Work out the finished part from the listing and answer in its coordinate system (mm). Face numbers are marked on the shaded views. A direction names the side the tool comes from. Coordinates: 2 decimals unless noted, no trailing zeros. Loops run counter-clockwise (first coordinate to the right, second up) from the corner with the lowest first, then second, coordinate; pieces in that order, holes last. Notation, with made-up numbers: (10, 60) -> (60, 60) arc R22 ccw to (60, 72) -> close; hole circle Ø1 at (43.25, 1.25). An arc over 180 degrees is marked (long way). Use a Markdown table: item, result. Add a question column.
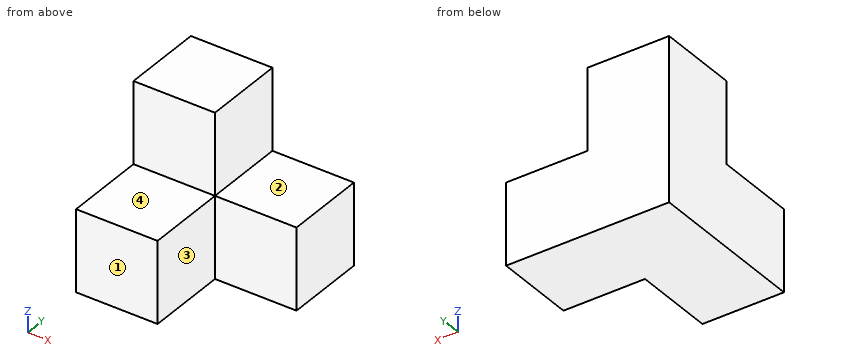
```python
from build123d import *

# Parameters (mm, degrees)
F0_W     = 19.05
F0_H     = 19.05
F1_DEPTH = 19.05
F2_W     = 19.05
F2_H     = 19.05
F3_DEPTH = 19.05


with BuildPart() as f1:
    # F0 (on Front) → F1 (new body)
    with BuildSketch(Plane.XZ):
        Rectangle(F0_W, F0_H)
        Polygon((28.575, -9.525), (9.525, -9.525), (-9.525, -9.525), (-9.525, -28.575), (28.575, -28.575), align=None)
    extrude(amount=F1_DEPTH)

    # F2 (on face) → F3 (join)
    with BuildSketch(Plane.XZ.offset(19.05)):
        with Locations((0, -19.05)):
            Rectangle(F2_W, F2_H)
    extrude(amount=F3_DEPTH)


solid = f1.part
```
Item 1: Section C-C (y = -25.5) is taken. Determine the outline of the cut face in (x, z) (3 decimals).
Item 2: Section A-A (z = -20.5) is taken. Determine the outline of the cut face in (x, y) (3 decimals).
Item 3: For the marked faces 1, 2, 3 and 4, determine the directions among +Z, -Z, +X, -X, +Y, -Y from which every point of the face is accessible in a straight line to the end or side of a thin tool.
Item 4: Given pin 1 (9.5 mm diameter, centred on x = 23.5, y = -9, fed in from +Z) (3 decimals); pin 2 (9.5 mm diameter, centred on x = -4.5, z = -4.5, fed in from -Y); pin 3 (9.5 mm diameter, centred on y = -7, z = 2, fed in from +X) (3 decimals), each flat-ended and moving along its own axis, determine where each tip first touches the part or whether it passes through.
Item 5: Find the intervals of material crossed by probe 1 along X at (y, z) = (-7.5, -2) (3 decimals); probe 2 along Y at (x, z) = (12, -10); probe 3 along Z at (x, y) = (22.5, -14.5) (3 decimals), in increasing order.
Item 6: Section B-B (y = -3) is taken. Determine the outline of the cut face in (x, z) (3 decimals), then the cut area to 3 significant figures.
Item 7: Section D-D (z = 1) is taken. Determine the outline of the cut face in (x, y) (3 decimals).
Output:
| question | item | result |
|---|---|---|
| 1 | outline | (-9.525, -28.575) -> (9.525, -28.575) -> (9.525, -9.525) -> (-9.525, -9.525) -> close |
| 2 | outline | (-9.525, -38.1) -> (9.525, -38.1) -> (9.525, -19.05) -> (28.575, -19.05) -> (28.575, 0) -> (-9.525, 0) -> close |
| 3 | face 1 | +Z, -Z, +X, -X, -Y |
| 3 | face 2 | +Z, +X, +Y, -Y |
| 3 | face 3 | +Z, -Z, +X, -Y |
| 3 | face 4 | +Z, +X, -X, -Y |
| 4 | pin 1 | stops at z = -9.525 |
| 4 | pin 2 | stops at y = -19.05 |
| 4 | pin 3 | stops at x = 9.525 |
| 5 | probe 1 | x = -9.525 to 9.525 |
| 5 | probe 2 | y = -19.05 to 0 |
| 5 | probe 3 | z = -28.575 to -9.525 |
| 6 | outline | (-9.525, -28.575) -> (28.575, -28.575) -> (28.575, -9.525) -> (9.525, -9.525) -> (9.525, 9.525) -> (-9.525, 9.525) -> close |
| 6 | area | 1,090 mm2 |
| 7 | outline | (-9.525, -19.05) -> (9.525, -19.05) -> (9.525, 0) -> (-9.525, 0) -> close |
